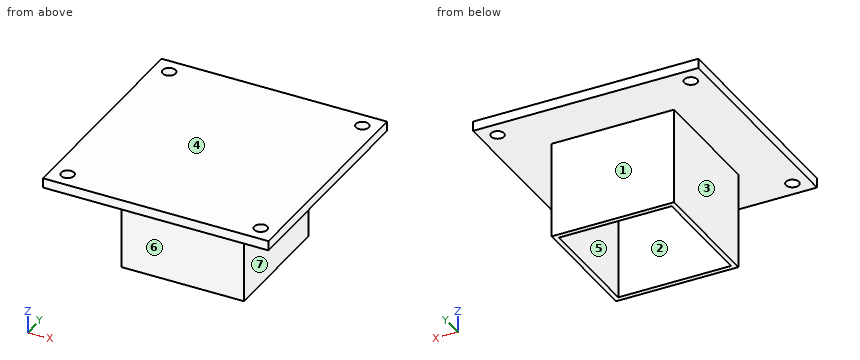
from build123d import *

# Parameters (mm, degrees)
SKETCH1_W           = 70
SKETCH1_H           = 70
BOSS_EXTRUDE1_DEPTH = 3
SKETCH3_R           = 2
CUT_EXTRUDE1_DEPTH  = 4
SKETCH5_W           = 38
SKETCH5_H           = 38
SKETCH5_W_2         = 35
SKETCH5_H_2         = 35
BOSS_EXTRUDE2_DEPTH = 30


with BuildPart() as part:
    # Sketch1 → Boss-Extrude1 (new body)
    with BuildSketch(Plane.XY):
        Rectangle(SKETCH1_W, SKETCH1_H)
    extrude(amount=BOSS_EXTRUDE1_DEPTH)

    # Sketch3 → Cut-Extrude1 (cut)
    with BuildSketch(Plane.XY.offset(3)):
        with Locations((-30, 30)):
            Circle(SKETCH3_R)
        with Locations((30, 30)):
            Circle(SKETCH3_R)
        with Locations((30, -30)):
            Circle(SKETCH3_R)
        with Locations((-30, -30)):
            Circle(SKETCH3_R)
    extrude(amount=-CUT_EXTRUDE1_DEPTH, mode=Mode.SUBTRACT)

    # Sketch5 → Boss-Extrude2 (add)
    with BuildSketch(Plane(origin=(0, 0, 0), x_dir=(-1, 0, 0), z_dir=(0, 0, -1))):
        Rectangle(SKETCH5_W, SKETCH5_H)
        Rectangle(SKETCH5_W_2, SKETCH5_H_2, mode=Mode.SUBTRACT)
    extrude(amount=BOSS_EXTRUDE2_DEPTH)


solid = part.part
Check sheet for the modelled part. Datum: model origin and axes. Units: mm. Face numbers are marked on the shaded views. A direction names the side the tool comes from. Give positions to 0.01 mm unless a question says otherwise; leave off trailing zeros. Write each loop counter-clockwise with the first axis right and the second up, starting at its lowest first coordinate (ties: lowest second). Pieces come first, ordered by that corner, then holes. Notation, with made-up numbers: M -19,2 L 18,2 A26 cw 18,41 Z; hole C 67,14 d3. An arc over 180 degrees is marked long. Use one line per item in the form item = value.
(1) Section check B-B on z = -17. Record the boundary of the cut face in (x, y).
Answer block:
outline = M -19,-19 L 19,-19 L 19,19 L -19,19 Z; hole M -17.5,-17.5 L 17.5,-17.5 L 17.5,17.5 L -17.5,17.5 Z
(2) Depth check by flat-ended pin: P1, Ø9, axis at x = 6, z = -13.5, coming from the +Y side; P2, Ø4, axis at x = -11, y = -11.5, coming from the -Z side; P3, Ø2, axis at y = -15.5, z = -23.5, coming from the +X side. Enter the tip coordinate at first touch or a pass-through.
Answer block:
P1 = 19
P2 = 0
P3 = 19
(3) Tool access check on the marked faces 1, 2, 3 and 4. Record the directions out of +Z, -Z, +X, -X, +Y, -Y that give a thin tool (end or side, any length) a straight path to the whole face; none if there is none.
Answer block:
face_1 = -Z, +X, -X, +Y
face_2 = -Z
face_3 = -Z, -X, +Y, -Y
face_4 = +Z, +X, -X, +Y, -Y
(4) Material ranges on line 1 along Y through (x, z) = (-30, 2); line 2 along Y through (x, z) = (-5, -14), recorded low to high.
Answer block:
line_1 = -35 to -32, -28 to 28, 32 to 35
line_2 = -19 to -17.5, 17.5 to 19
(5) Draft check along X on the marked faces 5, 6 and 7. Enter one of: pulls with the +X half, pulls with the -X half, needs draft (parallel to the pull), parting line crosses it, or undercut.
Answer block:
face_5 = undercut
face_6 = needs draft
face_7 = pulls with the +X half
(6) Section check A-A on x = 30. Record the boundary of the cut face in (y, z).
Answer block:
outline = M -35,0 L -32,0 L -32,3 L -35,3 Z; M -28,0 L 28,0 L 28,3 L -28,3 Z; M 32,0 L 35,0 L 35,3 L 32,3 Z
(7) Section check D-D on x = -13. Record the boundary of the cut face in (y, z).
Answer block:
outline = M -35,0 L -19,0 L -19,-30 L -17.5,-30 L -17.5,0 L 17.5,0 L 17.5,-30 L 19,-30 L 19,0 L 35,0 L 35,3 L -35,3 Z
